Geometry check sheet. Reference: drawing and pictorial views, mm from the part's lowest x, y, z. Give positions to 0.01 mm unless a question says otherwise; leave off trailing zeros. Write each loop counter-clockwise with the first axis right and the second up, starting at its lowest first coordinate (ties: lowest second). Pieces come first, ordered by that corner, then holes. Notation, with made-up numbers: (79.25, 63) - (137.25, 63) arc R22 ccw to (137.25, 76) - close; hole circle Ø2 at (46, 31). An arc over 180 degrees is marked (long way). Put each result on its own line as item: value.
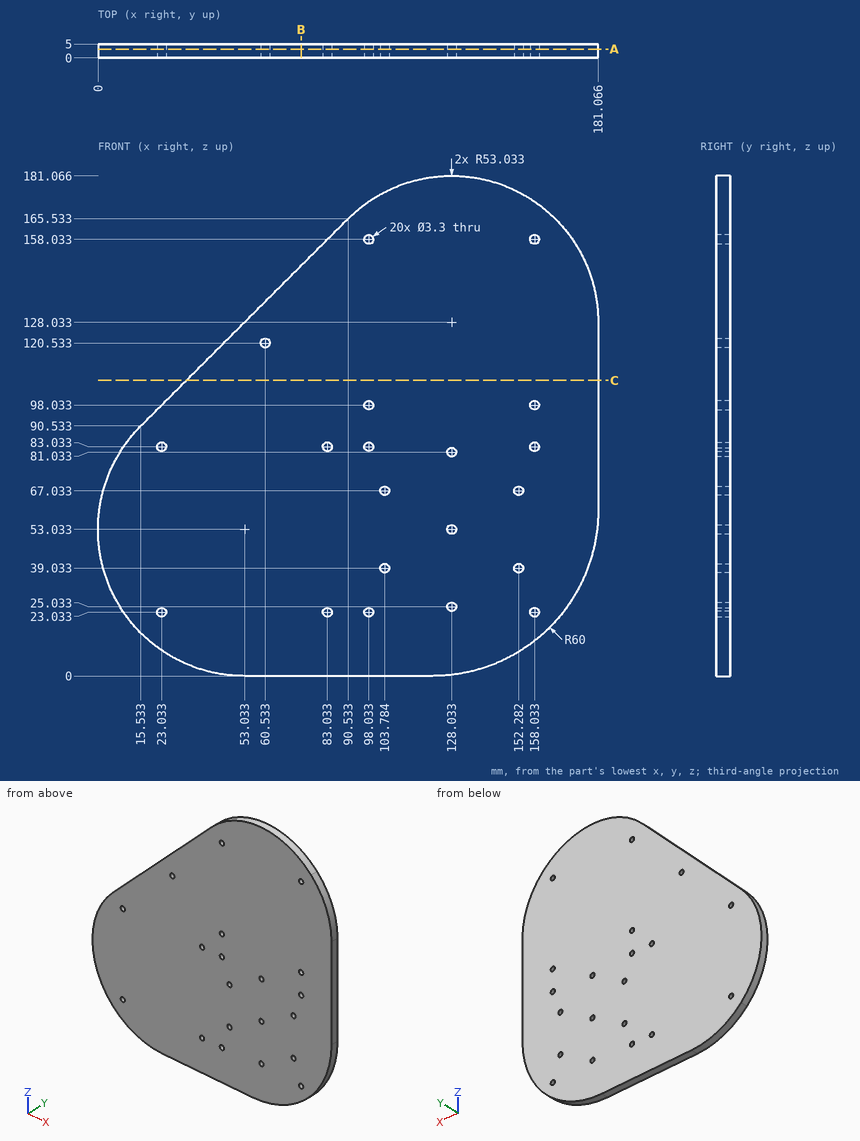
Q1. Section check A-A, the plane y = 3.15. Give the number of separate pieces and of enclosed holes in the cut face, plus the area to 3 significant figures.
Answers follow:
separate pieces: 1
enclosed holes: 20
area: 24,900 mm2
Q2. Go/stop test with flat-tipped pins: pin 1 Ø3 at (y, z) = (4.5, 160) entering from +X; pin 2 Ø1 at (x, y) = (129.5, 4) entering from -Z; pin 3 Ø3 at (x, z) = (80.5, 147.5) entering from -Y; pin 4 Ø3 at (x, y) = (53, 3.5) entering from +Z. Record where each tip stops, or that it passes through.
Answers follow:
pin 1: stops at x = 171.44
pin 2: stops at z = 0.53
pin 3: stops at y = 0
pin 4: stops at z = 129.5
Q3. Section check B-B, the plane x = 73.5. Record the cut outline in (y, z).
Answers follow:
outline: (0, 0) - (5, 0) - (5, 148.5) - (0, 148.5) - close
Q4. Section check C-C, the plane z = 107. Record the cut outline in (x, y).
Answers follow:
outline: (32, 0) - (181.07, 0) - (181.07, 5) - (32, 5) - close
Q5. Scan lines: line 1 along X through (y, z) = (1.5, 40) (1 decimal); line 2 along X through (y, z) = (4.1, 39) (1 decimal); line 3 along X through (y, z) = (2.4, 24) (1 decimal). Record each from-to range of solid material in increasing order.
Answers follow:
line 1: x = 1.6 to 102.4, 105.1 to 150.9, 153.6 to 177.6
line 2: x = 1.9 to 102.1, 105.4 to 150.6, 153.9 to 177.3
line 3: x = 8.7 to 21.7, 24.4 to 81.7, 84.4 to 96.7, 99.4 to 126.7, 129.3 to 156.7, 159.4 to 169.1
